from build123d import *

# Parameters (mm, degrees)
SKETCH1_W           = 100
SKETCH1_H           = 100
SKETCH1_R           = 7.5
SKETCH1_R_2         = 4
SKETCH1_W_2         = 4.1
SKETCH1_H_2         = 15
SKETCH1_W_3         = 15
SKETCH1_H_3         = 4.1
BOSS_EXTRUDE1_DEPTH = 4.1


with BuildPart() as part:
    # Sketch1 → Boss-Extrude1 (new body)
    with BuildSketch(Plane(origin=(0, 0, 0), x_dir=(1, 0, 0), z_dir=(0, 1, 0))):
        Rectangle(SKETCH1_W, SKETCH1_H)
        Circle(SKETCH1_R, mode=Mode.SUBTRACT)
        with Locations((-38.183766184, -38.183766184)):
            Circle(SKETCH1_R_2, mode=Mode.SUBTRACT)
        with Locations((-22.95, 37.5)):
            Rectangle(SKETCH1_W_2, SKETCH1_H_2, mode=Mode.SUBTRACT)
        with Locations((-37.5, 22.95)):
            Rectangle(SKETCH1_W_3, SKETCH1_H_3, mode=Mode.SUBTRACT)
        with Locations((37.5, -22.95)):
            Rectangle(SKETCH1_W_3, SKETCH1_H_3, mode=Mode.SUBTRACT)
        with Locations((22.95, -37.5)):
            Rectangle(SKETCH1_W_2, SKETCH1_H_2, mode=Mode.SUBTRACT)
        with Locations((37.5, 22.95)):
            Rectangle(SKETCH1_W_3, SKETCH1_H_3, mode=Mode.SUBTRACT)
        with Locations((-37.5, -22.95)):
            Rectangle(SKETCH1_W_3, SKETCH1_H_3, mode=Mode.SUBTRACT)
        with Locations((22.95, 37.5)):
            Rectangle(SKETCH1_W_2, SKETCH1_H_2, mode=Mode.SUBTRACT)
        with Locations((-22.95, -37.5)):
            Rectangle(SKETCH1_W_2, SKETCH1_H_2, mode=Mode.SUBTRACT)
        with Locations((0, 39.95)):
            Rectangle(SKETCH1_W_3, SKETCH1_H_3, mode=Mode.SUBTRACT)
        with Locations((0, -39.95)):
            Rectangle(SKETCH1_W_3, SKETCH1_H_3, mode=Mode.SUBTRACT)
        with Locations((39.95, 0)):
            Rectangle(SKETCH1_W_2, SKETCH1_H_2, mode=Mode.SUBTRACT)
        with Locations((-39.95, 0)):
            Rectangle(SKETCH1_W_2, SKETCH1_H_2, mode=Mode.SUBTRACT)
    extrude(amount=BOSS_EXTRUDE1_DEPTH)


solid = part.part
Check sheet for the modelled part. Datum: model origin and axes. Units: mm. Give positions to 0.01 mm unless a question says otherwise; leave off trailing zeros. Order: outer loops, then holes, each group sorted by start corner. A loop starts at its lowest first (then second) coordinate and runs counter-clockwise, first axis right, second up. Notation, with made-up numbers: (15.5, 74.5) - (29.5, 74.5) arc R8 ccw to (29.5, 87.5) - close; hole circle Ø11 at (62, 72.25). An arc over 180 degrees is marked (long way). Answer as CSV lines item,"result".
1. Section check A-A (z = 0). Record the boundary of the cut face in (x, y).
Result sheet:
outline,"(-50, 0) - (-42, 0) - (-42, 4.1) - (-50, 4.1) - close; (-37.9, 0) - (-7.5, 0) - (-7.5, 4.1) - (-37.9, 4.1) - close; (7.5, 0) - (37.9, 0) - (37.9, 4.1) - (7.5, 4.1) - close; (42, 0) - (50, 0) - (50, 4.1) - (42, 4.1) - close"
2. Section check C-C (z = -32). Record the boundary of the cut face in (x, y), then the cut area to 3 significant figures.
Result sheet:
outline,"(-50, 0) - (-25, 0) - (-25, 4.1) - (-50, 4.1) - close; (-20.9, 0) - (20.9, 0) - (20.9, 4.1) - (-20.9, 4.1) - close; (25, 0) - (50, 0) - (50, 4.1) - (25, 4.1) - close"
area,"376 mm²"
3. Scan lines: probe 1 along Z at (x, y) = (24, 0.45); probe 2 along Z at (x, y) = (-43.5, 1.9). Record each from-to range of solid material in increasing order. Write a range as from..to.
Result sheet:
probe 1,"-50..-45, -30..30, 45..50"
probe 2,"-50..-25, -20.9..20.9, 25..50"
4. Mould release check, pull along X, two halves, no side actions. Record for faces 1 (the face through (-50, 2, 1)), 2 (the face through (-1, 2, -50)), 3 (the face through (7.5, 2, -40)): released by +X, released by -X, zero draft, split by the parting line, or undercut.
Result sheet:
face 1,"released by -X"
face 2,"zero draft"
face 3,"undercut"
5. Section check B-B (x = 0). Record the boundary of the cut face in (y, z).
Result sheet:
outline,"(0, -50) - (4.1, -50) - (4.1, -42) - (0, -42) - close; (0, -37.9) - (4.1, -37.9) - (4.1, -7.5) - (0, -7.5) - close; (0, 7.5) - (4.1, 7.5) - (4.1, 37.9) - (0, 37.9) - close; (0, 42) - (4.1, 42) - (4.1, 50) - (0, 50) - close"
6. Section check D-D (y = 1.1). State how many separate pieces and enclosed holes the cut face has, then the cut area to 4 significant figures.
Result sheet:
separate pieces,"1"
enclosed holes,"14"
area,"9,035 mm²"
